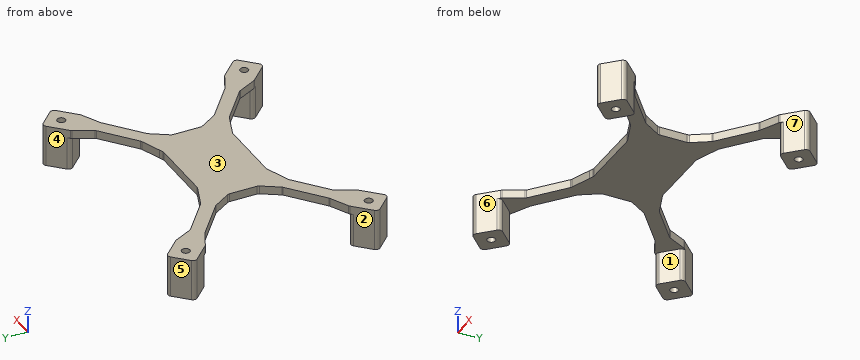
```python
from build123d import *

# Parameters (mm, degrees)
BOSS_EXTRUDE1_DEPTH   = 15
BOSS_EXTRUDE1_2_DEPTH = 15
BOSS_EXTRUDE1_3_DEPTH = 15
BOSS_EXTRUDE1_4_DEPTH = 15
BOSS_EXTRUDE2_DEPTH   = 3
F_2_CLEARANCE_HOLE1_D = 2.9464
FILLET2_R             = 1.5
FILLET3_R             = 1.5


with BuildPart() as part:
    # Sketch1 → Boss-Extrude1 (new body)
    with BuildSketch(Plane.XY):
        Polygon((-51.196067812, 33.16), (-44.125, 40.231067812), (-37.053932188, 33.16), (-44.125, 26.088932188), align=None)
    extrude(amount=BOSS_EXTRUDE1_DEPTH)



with BuildPart() as body_2:
    # Sketch1 → Boss-Extrude1 2 (new body)
    with BuildSketch(Plane.XY):
        Polygon((44.125, 26.088932188), (37.053932188, 33.16), (44.125, 40.231067812), (51.196067812, 33.16), align=None)
    extrude(amount=BOSS_EXTRUDE1_2_DEPTH)


with BuildPart() as body_3:
    # Sketch1 → Boss-Extrude1 3 (new body)
    with BuildSketch(Plane.XY):
        Polygon((37.053932188, -33.16), (44.125, -26.088932188), (51.196067812, -33.16), (44.125, -40.231067812), align=None)
    extrude(amount=BOSS_EXTRUDE1_3_DEPTH)


with BuildPart() as body_4:
    # Sketch1 → Boss-Extrude1 4 (new body)
    with BuildSketch(Plane.XY):
        Polygon((-44.125, -40.231067812), (-51.196067812, -33.16), (-44.125, -26.088932188), (-37.053932188, -33.16), align=None)
    extrude(amount=BOSS_EXTRUDE1_4_DEPTH)


with BuildPart() as part_1:
    add(part.part)

    add(body_2.part)  # Boss-Extrude2 merges body 2

    add(body_3.part)  # Boss-Extrude2 merges body 3

    add(body_4.part)  # Boss-Extrude2 merges body 4
    # Sketch2 → Boss-Extrude2 (add)
    with BuildSketch(Plane.XY.offset(15)):
        Polygon((-16.839511506, 12.5), (16.839511506, 12.5), (33.509317925, 26.098012545), (37.053932188, 33.16), (44.125, 26.088932188), (37.063012545, 22.544317925), (20, 8.625556495), (20, -8.625556495), (37.063012545, -22.544317925), (44.125, -26.088932188), (37.053932188, -33.16), (33.509317925, -26.098012545), (16.839511506, -12.5), (-16.839511506, -12.5), (-33.509317925, -26.098012545), (-37.053932188, -33.16), (-44.125, -26.088932188), (-37.063012545, -22.544317925), (-20, -8.625556495), (-20, 8.625556495), align=None)
        Polygon((-13.695257257, 13.144844299), (-21.07904964, 15.95830607), (-16.839511506, 12.5), (-12.002895034, 12.5), align=None)
        Polygon((-16.839511506, 12.5), (-20, 8.625556495), (-37.063012545, 22.544317925), (-44.125, 26.088932188), (-37.053932188, 33.16), (-33.509317925, 26.098012545), align=None)
        Polygon((-20, 8.625556495), (-24.239538134, 12.083862565), (-20, 5.415858854), align=None)
        Polygon((-20, -8.625556495), (-20, -5.415858854), (-24.239538134, -12.083862565), align=None)
        Polygon((-16.839511506, -12.5), (-21.07904964, -15.95830607), (-13.695257257, -13.144844299), (-12.002895034, -12.5), align=None)
        Polygon((16.839511506, -12.5), (12.002895034, -12.5), (13.695257257, -13.144844299), (21.07904964, -15.95830607), align=None)
        Polygon((24.239538134, -12.083862565), (20, -5.415858854), (20, -8.625556495), align=None)
        Polygon((20, 5.415858854), (24.239538134, 12.083862565), (20, 8.625556495), align=None)
        Polygon((13.695257257, 13.144844299), (12.002895034, 12.5), (16.839511506, 12.5), (21.07904964, 15.95830607), align=None)
    extrude(amount=-BOSS_EXTRUDE2_DEPTH)

    # #2 Clearance Hole1 (through all)
    with Locations(Plane(origin=(0, 0, 0), x_dir=(-1, 0, 0), z_dir=(0, 0, -1))):
        with Locations((-44.125, 33.16), (44.125, 33.16), (44.125, -33.16), (-44.125, -33.16)):
            Hole(F_2_CLEARANCE_HOLE1_D / 2)

    # Fillet2
    fillet2_edges = [part_1.edges().sort_by_distance(p)[0] for p in [
        (37.053932188, 33.16, 6),
        (44.125, 26.088932188, 6),
        (51.196067812, 33.16, 7.5),
        (44.125, 40.231067812, 7.5),
        (44.125, -26.088932188, 6),
        (37.053932188, -33.16, 6),
        (44.125, -40.231067812, 7.5),
        (51.196067812, -33.16, 7.5),
        (-44.125, -40.231067812, 7.5),
        (-37.053932188, -33.16, 6),
        (-44.125, -26.088932188, 6),
        (-51.196067812, -33.16, 7.5),
        (-37.053932188, 33.16, 6),
        (-44.125, 26.088932188, 6),
        (-51.196067812, 33.16, 7.5),
        (-44.125, 40.231067812, 7.5),
    ]]
    fillet(fillet2_edges, radius=FILLET2_R)

    # Fillet3
    fillet3_edges = [part_1.edges().sort_by_distance(p)[0] for p in [
        (20, 5.415858854, 13.5),
        (20, -5.415858854, 13.5),
        (24.239538134, -12.083862565, 13.5),
        (37.063012545, -22.544317925, 13.5),
        (44.125, -26.088932188, 13.5),
        (37.053932188, -33.16, 13.5),
        (33.509317925, -26.098012545, 13.5),
        (21.07904964, -15.95830607, 13.5),
        (12.002895034, -12.5, 13.5),
        (-12.002895034, -12.5, 13.5),
        (-21.07904964, -15.95830607, 13.5),
        (-33.509317925, -26.098012545, 13.5),
        (-37.053932188, -33.16, 13.5),
        (-44.125, -26.088932188, 13.5),
        (-37.063012545, -22.544317925, 13.5),
        (-24.239538134, -12.083862565, 13.5),
        (-20, -5.415858854, 13.5),
        (-20, 5.415858854, 13.5),
        (-24.239538134, 12.083862565, 13.5),
        (-37.063012545, 22.544317925, 13.5),
        (-33.509317925, 26.098012545, 13.5),
        (-21.07904964, 15.95830607, 13.5),
        (-12.002895034, 12.5, 13.5),
        (12.002895034, 12.5, 13.5),
        (21.07904964, 15.95830607, 13.5),
        (33.509317925, 26.098012545, 13.5),
        (37.053932188, 33.16, 13.5),
        (44.125, 26.088932188, 13.5),
        (37.063012545, 22.544317925, 13.5),
        (24.239538134, 12.083862565, 13.5),
        (-37.053932188, 33.16, 13.5),
        (-44.125, 26.088932188, 13.5),
    ]]
    fillet(fillet3_edges, radius=FILLET3_R)


solid = part_1.part
```
Verification items for the finished model (mm, model axes). Face numbers are marked on the shaded views. A direction names the side the tool comes from. Give positions to 0.01 mm unless a question says otherwise; leave off trailing zeros. Loops run counter-clockwise (first coordinate to the right, second up) from the corner with the lowest first, then second, coordinate; pieces in that order, holes last. Notation, with made-up numbers: M 7,13 L 21,13 A22 cw 21,28 Z; hole C 34.5,6 d4. An arc over 180 degrees is marked long. Return JSON: item names as keys, results as strings.
1) Gauge pin test, flat ends, axial feed: P1, Ø2.5, axis at x = -44.125, y = 33.16, coming from the -Z side; P2, Ø1, axis at y = -15.5, z = 12, coming from the +X side; P3, Ø2.5, axis at y = 1.5, z = 13.5, coming from the -X side; P4, Ø1.5, axis at x = -3, z = 13.5, coming from the +Y side. Record the tip position at first contact, or that the pin passes through.
Findings:
{"P1": "passes through", "P2": "stops at x = 29.04", "P3": "stops at x = -20", "P4": "stops at y = 12.5"}
2) Mould release check, pull along Y, two halves, no side actions. Record for the marked faces 5, 6 and 7: released by +Y, released by -Y, zero draft, split by the parting line, or undercut.
Findings:
{"face 5": "released by +Y", "face 6": "released by -Y", "face 7": "undercut"}
3) Section check C-C, the plane x = 2. Enter the section's corners in (y, z), and give its area (3 significant figures).
Findings:
{"outline": "M -12.5,12 L 12.5,12 L 12.5,15 L -12.5,15 Z", "area": "75.0 mm2"}
4) Section check A-A, the plane z = 1.75. Count the separate pieces of the cut face and the enclosed holes in it, and give its area (3 significant figures).
Findings:
{"separate pieces": "4", "enclosed holes": "4", "area": "365 mm2"}
5) Section check B-B, the plane y = 24. Enter the section's corners in (x, z).
Findings:
{"outline": "M -39.96,12 L -30.94,12 L -30.94,15 L -39.96,15 Z; M 30.94,12 L 39.96,12 L 39.96,15 L 30.94,15 Z"}
6) Tool access check on the marked faces 1, 2, 3 and 4. Record the directions out of +Z, -Z, +X, -X, +Y, -Y that give a thin tool (end or side, any length) a straight path to the whole face; none if there is none.
Findings:
{"face 1": "-Z", "face 2": "+Z, -Z, -X", "face 3": "+Z, +X, -X, +Y, -Y", "face 4": "+Z, -Z, +Y"}
7) Material ranges on L1, parallel to Z at x = -17.5, y = -4.5; L2, parallel to X at y = -1.5, z = 12.75; L3, parallel to Y at x = 40, z = 11.25, recorded low to high. Write a range as [from, to].
Findings:
{"L1": "z = [12, 15]", "L2": "x = [-20, 20]", "L3": "y = [-36.11, -30.21], [30.21, 36.11]"}
